For this review, take the finished solid that the model builds, in its own axes (mm). Coordinates: 2 decimals unless noted, no trailing zeros. Answer as a JSON object with one key per item and string values. Group by question number.
1) For pin 1 (3 mm diameter, centred on x = 156.95, y = 40.91, fed in from -Z); pin 2 (3 mm diameter, centred on y = 26.5, z = 0.5, fed in from +X), all flat-tipped, find the tip position at first contact; note any pin that passes through.
2) Add section A-A, the plane z = 2. Count the separate pieces of the cut face and the enclosed holes in it, then the cut area to 3 significant figures.
3) Wall thickness on L1, parallel to Y at x = -36, z = 0.5; L2, parallel to X at y = 69, z = 5.5; L3, parallel to X at y = 102, z = 4.25: over which ranges is each line inside the solid? List them lowest first.
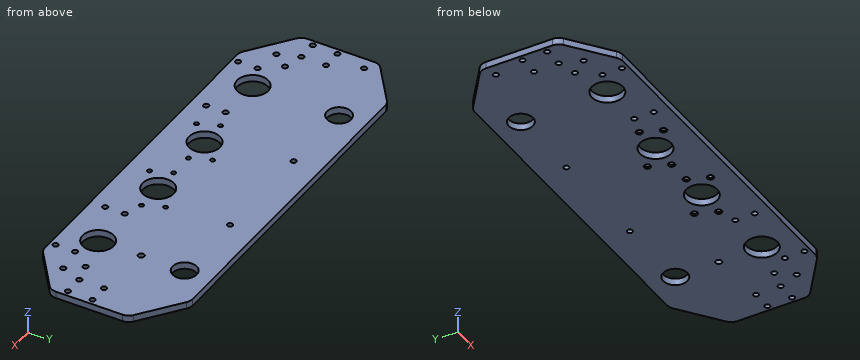
from build123d import *

# Parameters (mm, degrees)
SALIENTE_EXTRUIR1_DEPTH    = 6.35
REDONDEO1_R                = 10
CROQUIS2_R                 = 14.345
CORTAR_EXTRUIR1_DEPTH      = 10
CORTAR_EXTRUIR2_DEPTH      = 241.691916085
CORTAR_EXTRUIR2_DEPTH_BACK = 241.691916085
CROQUIS8_R                 = 14.345
CROQUIS8_R_2               = 2.01
CROQUIS8_R_3               = 2.02
CHAFL_N3_SIZE              = 1
CROQUIS9_R                 = 11.1125
CORTAR_EXTRUIR3_DEPTH      = 10
CROQUIS10_R                = 2.5
CROQUIS10_R_2              = 2.843216267
CORTAR_EXTRUIR4_DEPTH      = 10
CROQUIS11_R                = 2.5
CORTAR_EXTRUIR5_DEPTH      = 10


with BuildPart() as part:
    # Croquis1 → Saliente-Extruir1 (new body)
    with BuildSketch(Plane.XY):
        Polygon((155, 0), (-155, 0), (-198.126317543, 32.49801125), (-198.126317543, 104.023922026), (-155, 136.521933277), (155, 136.521933277), (198.126317543, 104.023922026), (198.126317543, 32.49801125), align=None)
    extrude(amount=SALIENTE_EXTRUIR1_DEPTH)

    # Redondeo1
    redondeo1_edges = [part.edges().sort_by_distance(p)[0] for p in [
        (198.126317543, 32.49801125, 3.175),
        (155, 0, 3.175),
        (-155, 0, 3.175),
        (-198.126317543, 32.49801125, 3.175),
        (198.126317543, 104.023922026, 3.175),
        (155, 136.521933277, 3.175),
        (-155, 136.521933277, 3.175),
        (-198.126317543, 104.023922026, 3.175),
    ]]
    fillet(redondeo1_edges, radius=REDONDEO1_R)

    # Croquis2 → Cortar-Extruir1 (cut)
    with BuildSketch(Plane.XY.offset(6.35)):
        with Locations((-121.592420883, 31.75)):
            Circle(CROQUIS2_R)
        with Locations((121.592420883, 31.75)):
            Circle(CROQUIS2_R)
    extrude(amount=-CORTAR_EXTRUIR1_DEPTH, mode=Mode.SUBTRACT)

    # Croquis8 → Cortar-Extruir2 (cut, two sides: drawn at the far end of the back side and taken through both)
    with BuildSketch(Plane.XY.offset(6.35).offset(-CORTAR_EXTRUIR2_DEPTH_BACK)):
        with Locations((-36.442420883, 37.2)):
            Circle(CROQUIS8_R)
        with Locations((36.442420883, 37.2)):
            Circle(CROQUIS8_R)
        with Locations((12.057209477, 37.2)):
            Circle(CROQUIS8_R_2)
        with Locations((19.496697235, 19.239487758)):
            Circle(CROQUIS8_R_2)
        with Locations((62.857209477, 37.2)):
            Circle(CROQUIS8_R_2)
        with Locations((55.417721719, 55.160512242)):
            Circle(CROQUIS8_R_2)
        with Locations((-18.48190864, 55.160512242)):
            Circle(CROQUIS8_R_3)
        with Locations((-11.042420883, 37.2)):
            Circle(CROQUIS8_R_3)
        with Locations((-54.402933125, 19.239487758)):
            Circle(CROQUIS8_R_3)
        with Locations((-61.842420883, 37.2)):
            Circle(CROQUIS8_R_3)
        with Locations((-121.592420883, 31.75)):
            Circle(CROQUIS8_R)
    extrude(amount=CORTAR_EXTRUIR2_DEPTH + CORTAR_EXTRUIR2_DEPTH_BACK, mode=Mode.SUBTRACT)

    # Chaflán3
    chafl_n3_edges = [part.edges().sort_by_distance(p)[0] for p in [
        (-63.862420883, 37.2, 0),
        (10.047209477, 37.2, 0),
        (-13.062420883, 37.2, 0),
        (-20.50190864, 55.160512242, 0),
        (-56.422933125, 19.239487758, 0),
        (53.407721719, 55.160512242, 0),
        (60.847209477, 37.2, 0),
        (17.486697235, 19.239487758, 0),
    ]]
    chamfer(chafl_n3_edges, length=CHAFL_N3_SIZE)

    # Croquis9 → Cortar-Extruir3 (cut)
    with BuildSketch(Plane(origin=(0, 0, 0), x_dir=(-1, 0, 0), z_dir=(0, 0, -1))):
        with Locations((-121.592420883, 111.521933277)):
            Circle(CROQUIS9_R)
        with Locations(Location((121.592420883, 111.521933277, 0), (0, 0, 180))):
            Circle(CROQUIS9_R)
    extrude(amount=-CORTAR_EXTRUIR3_DEPTH, mode=Mode.SUBTRACT)

    # Croquis10 → Cortar-Extruir4 (cut)
    with BuildSketch(Plane(origin=(0, 0, 0), x_dir=(-1, 0, 0), z_dir=(0, 0, -1))):
        with Locations((-50, 111.521933277)):
            Circle(CROQUIS10_R)
        with Locations(Location((50, 111.521933277, 0), (0, 0, 180))):
            Circle(CROQUIS10_R)
        with Locations((-121.592420883, 71.461933277)):
            Circle(CROQUIS10_R_2)
        with Locations((186.592420883, 96.521933277)):
            Circle(CROQUIS10_R)
    extrude(amount=-CORTAR_EXTRUIR4_DEPTH, mode=Mode.SUBTRACT)

    # Croquis11 → Cortar-Extruir5 (cut)
    with BuildSketch(Plane.XY.offset(6.35)):
        with Locations((-143.654046805, 23.35)):
            Circle(CROQUIS11_R)
        with Locations((-143.654046805, 5.35)):
            Circle(CROQUIS11_R)
        with Locations((-79.522420883, 31.5)):
            Circle(CROQUIS11_R)
        with Locations((-79.522420883, 13.5)):
            Circle(CROQUIS11_R)
        with Locations((143.654046805, 5.35)):
            Circle(CROQUIS11_R)
        with Locations((143.654046805, 23.35)):
            Circle(CROQUIS11_R)
        with Locations((79.522420883, 13.5)):
            Circle(CROQUIS11_R)
        with Locations((79.522420883, 31.5)):
            Circle(CROQUIS11_R)
        with Locations((-174.776317543, 45.483827331)):
            Circle(CROQUIS11_R)
        with Locations((-192.776317543, 45.483827331)):
            Circle(CROQUIS11_R)
        with Locations((-174.776317543, 68.260966638)):
            Circle(CROQUIS11_R)
        with Locations((-192.776317543, 68.260966638)):
            Circle(CROQUIS11_R)
        with Locations((174.776317543, 45.483827331)):
            Circle(CROQUIS11_R)
        with Locations((192.776317543, 45.483827331)):
            Circle(CROQUIS11_R)
        with Locations((192.776317543, 68.260966638)):
            Circle(CROQUIS11_R)
        with Locations((174.776317543, 68.260966638)):
            Circle(CROQUIS11_R)
        with Locations((-156.951159176, 40.912577131)):
            Circle(CROQUIS11_R)
        with Locations((-167.783829593, 26.537137951)):
            Circle(CROQUIS11_R)
        with Locations((167.783829593, 26.537137951)):
            Circle(CROQUIS11_R)
        with Locations((156.951159176, 40.912577131)):
            Circle(CROQUIS11_R)
    extrude(amount=-CORTAR_EXTRUIR5_DEPTH, mode=Mode.SUBTRACT)


solid = part.part
Output values:
{
 "1": {"pin 1": "passes through", "pin 2": "stops at x = 192.16"},
 "2": {"separate pieces": "1", "enclosed holes": "38", "area": "47,300 mm²"},
 "3": {"L1": "y = 0 to 22.86, 51.54 to 136.52", "L2": "x = -198.13 to -195.16, -190.39 to -177.16, -172.39 to 120.17, 123.01 to 172.39, 177.16 to 190.39, 195.16 to 198.13", "L3": "x = -197.68 to -127.32, -115.86 to 115.86, 127.32 to 197.68"}
}
